from build123d import *

# Parameters (mm, degrees)
EXTRUDE_1_DEPTH = 50
FILLET_1_R      = 3


with BuildPart() as part:
    # 草图2 → 凸台-拉伸1 (new body)
    with BuildSketch(Plane.XY):
        with BuildLine():
            Line((-200.898692044, 0), (-175, 0))
            ThreePointArc((-175, 0), (-172.9897341, 1.547802854), (-170.96577925, 3.077662138))
            Line((-170.96577925, 3.077662138), (-170.96577925, 42.722835601))
            ThreePointArc((-170.96577925, 42.722835601), (-153.932084993, 51.775484786), (-137.172282431, 42.225290265))
            Line((-137.172282431, 42.225290265), (-137.172282431, 24.846777263))
            ThreePointArc((-137.172282431, 24.846777263), (-130.71526297, 28.281929654), (-124.172282431, 31.55038157))
            Line((-124.172282431, 31.55038157), (-124.172282431, 40.001262339))
            ThreePointArc((-124.172282431, 40.001262339), (-112.742884956, 52.455330358), (-99.355672794, 42.134599408))
            ThreePointArc((-99.355672794, 42.134599408), (0, 60), (99.355672794, 42.134599408))
            ThreePointArc((99.355672794, 42.134599408), (112.742884956, 52.455330358), (124.172282431, 40.001262339))
            Line((124.172282431, 40.001262339), (124.172282431, 31.55038157))
            ThreePointArc((124.172282431, 31.55038157), (130.71526297, 28.281929654), (137.172282431, 24.846777263))
            Line((137.172282431, 24.846777263), (137.172282431, 42.225290265))
            ThreePointArc((137.172282431, 42.225290265), (153.932084993, 51.775484786), (170.96577925, 42.722835601))
            Line((170.96577925, 42.722835601), (170.96577925, 3.077662138))
            ThreePointArc((170.96577925, 3.077662138), (172.9897341, 1.547802854), (175, 0))
            Line((175, 0), (200.898692044, 0))
            Line((200.898692044, 0), (250, 70))
            ThreePointArc((250, 70), (0, 80), (-250, 70))
            Line((-250, 70), (-200.898692044, 0))
        make_face()
        with BuildLine():
            Line((-175, 0), (-158.179750074, 0))
            ThreePointArc((-158.179750074, 0), (0, 50), (158.179750074, 0))
            Line((158.179750074, 0), (175, 0))
            ThreePointArc((175, 0), (0, 60), (-175, 0))
        make_face()
    extrude(amount=EXTRUDE_1_DEPTH)

    # 圆角1
    fillet_1_edges = [part.edges().sort_by_distance(p)[0] for p in [
        (137.172282431, 24.846777263, 25),
        (170.96577925, 3.077662138, 25),
        (170.96577925, 42.722835601, 25),
        (137.172282431, 42.225290265, 25),
        (124.172282431, 31.55038157, 25),
        (99.355672794, 42.134599408, 25),
        (-99.355672794, 42.134599408, 25),
        (-124.172282431, 31.55038157, 25),
        (-137.172282431, 24.846777263, 25),
        (-137.172282431, 42.225290265, 25),
        (-170.96577925, 42.722835601, 25),
        (-170.96577925, 3.077662138, 25),
    ]]
    fillet(fillet_1_edges, radius=FILLET_1_R)


solid = part.part
Model file for the job. Use its own axes, mm. A direction names the side the tool comes from. Give positions to 0.01 mm unless a question says otherwise; leave off trailing zeros. Order: outer loops, then holes, each group sorted by start corner. A loop starts at its lowest first (then second) coordinate and runs counter-clockwise, first axis right, second up. Notation, with made-up numbers: (-36.5, 80.5) - (8.5, 80.5) arc R17 cw to (8.5, 106.5) - close; hole circle Ø6 at (-22.75, 29). An arc over 180 degrees is marked (long way). Write item = value, one per line. Start each with the question number.
1. Cut at A-A, the plane y = 15. List the corners of the cut face in (x, z), and give its area (3 significant figures).
2. Probe line 1 along X through (y, z) = (7, 21.5); line 2 along X through (y, z) = (24, 18); line 3 along Y through (x, z) = (-2, 14). List the from-to ranges inside material, lowest first.
3. Drop flat-ended pins along their axis: P1, Ø1, axis at x = -80, y = 53.5, coming from the -Z side; P2, Ø3, axis at x = 135, z = 9.5, coming from the +Y side; P3, Ø5, axis at y = 72, z = 36, coming from the -X side; P4, Ø1.5, axis at y = 57.5, z = 18, coming from the -X side. Give the stop position or say it passes through.
4. Cut at C-C, the plane z = 33.5. State how many separate pieces and enclosed holes the cut face has, and give its area (3 significant figures).
5. Cut at D-D, the plane x = 49. List the corners of the cut face in (y, z).
6. Cut at B-B, the plane x = 146.5. List the corners of the cut face in (y, z).
7. Two-plate mould, pull along Y, no slides. Class faces 1 (the flat face through (-170.966, 25, 25)), 2 (the flat face through (-3, 58, 0)), 3 (the cylindrical face through (111.13, 37.46, 24.65)), 4 (the flat face through (179, 0, 25)): pulls with the +Y half, pulls with the -Y half, needs draft (parallel to the pull), parting line crosses it, or undercut.
8. Which spindle directions (+Z, -Z, +X, -X, +Y, -Y) get a long thin tool onto all of the face, cutting with end or side? Do faces 5 (the cylindrical face through (-154.173, 51.778, 24.65)), 6 (the flat face through (-3, 58, 50)). Say none if no direction does.
Taken from the geometry:
q1.outline = (-211.42, 0) - (-170.97, 0) - (-170.97, 50) - (-211.42, 50) - close; (-153.77, 0) - (-134.31, 0) - (-134.31, 50) - (-153.77, 50) - close; (134.31, 0) - (153.77, 0) - (153.77, 50) - (134.31, 50) - close; (170.97, 0) - (211.42, 0) - (211.42, 50) - (170.97, 50) - close
q1.area = 5,990 mm²
q2.line_1 = -205.81 to -170.21, -165.6 to -147.71, 147.71 to 165.6, 170.21 to 205.81
q2.line_2 = -217.73 to -170.97, -138.7 to -116.77, 116.77 to 138.7, 170.97 to 217.73
q2.line_3 = 49.99 to 80
q3.P1 = 0
q3.P2 = 77.15
q3.P3 = -250
q3.P4 = -241.76
q4.separate_pieces = 1
q4.enclosed_holes = 4
q4.area = 21,200 mm²
q5.outline = (45.6, 0) - (79.62, 0) - (79.62, 50) - (45.6, 50) - close
q6.outline = (7.77, 0) - (19.5, 0) - (19.5, 50) - (7.77, 50) - close; (50.22, 0) - (76.57, 0) - (76.57, 50) - (50.22, 50) - close
q7.face_1 = undercut
q7.face_2 = needs draft
q7.face_3 = undercut
q7.face_4 = pulls with the -Y half
q8.face_5 = +Z, -Z
q8.face_6 = +Z, +X, -X, +Y, -Y
